from build123d import *

# Parameters (mm, degrees)
SKETCH1_W           = 20
SKETCH1_H           = 10
BOSS_EXTRUDE1_DEPTH = 20.5
SKETCH5_W           = 16
SKETCH5_H           = 12.5
BOSS_EXTRUDE2_DEPTH = 8
SKETCH2_R           = 5.1
CUT_EXTRUDE3_DEPTH  = 10
SKETCH6_W           = 5.5
SKETCH6_H           = 20
CUT_EXTRUDE4_DEPTH  = 8
SKETCH7_W           = 2.2
SKETCH7_H           = 2.2
CUT_EXTRUDE5_DEPTH  = 3
FILLET1_R           = 2


with BuildPart() as part:
    # Sketch1 → Boss-Extrude1 (new body)
    with BuildSketch(Plane.YZ):
        Rectangle(SKETCH1_W, SKETCH1_H)
    extrude(amount=BOSS_EXTRUDE1_DEPTH)

    # Sketch5 → Boss-Extrude2 (add)
    with BuildSketch(Plane(origin=(0, 0, 0), x_dir=(0, 1, 0), z_dir=(0, 0, 1))):
        with Locations((0, -12.25)):
            Rectangle(SKETCH5_W, SKETCH5_H)
    extrude(amount=BOSS_EXTRUDE2_DEPTH)

    # Sketch2 → Cut-Extrude3 (cut)
    with BuildSketch(Plane.YZ):
        Circle(SKETCH2_R)
    extrude(amount=CUT_EXTRUDE3_DEPTH, mode=Mode.SUBTRACT)

    # Sketch6 → Cut-Extrude4 (cut)
    with BuildSketch(Plane(origin=(0, 0, -5), x_dir=(1, 0, 0), z_dir=(0, 0, -1))):
        with Locations((17.75, 0)):
            Rectangle(SKETCH6_W, SKETCH6_H)
    extrude(amount=-CUT_EXTRUDE4_DEPTH, mode=Mode.SUBTRACT)

    # Sketch7 → Cut-Extrude5 (cut)
    with BuildSketch(Plane.YZ.offset(15)):
        with Locations((6, 0)):
            Rectangle(SKETCH7_W, SKETCH7_H)
        with Locations((-6, 0)):
            Rectangle(SKETCH7_W, SKETCH7_H)
    extrude(amount=-CUT_EXTRUDE5_DEPTH, mode=Mode.SUBTRACT)

    # Fillet1
    fillet1_edges = [part.edges().sort_by_distance(p)[0] for p in [
        (7.5, -10, -5),
        (7.5, 10, -5),
    ]]
    fillet(fillet1_edges, radius=FILLET1_R)


solid = part.part
Part model, mm, in its own coordinate system. A direction names the side the tool comes from. Give positions to 0.01 mm unless a question says otherwise; leave off trailing zeros. Loops run counter-clockwise (first coordinate to the right, second up) from the corner with the lowest first, then second, coordinate; pieces in that order, holes last. Notation, with made-up numbers: (40, 37) -> (62, 37) arc R19 ccw to (62, 60) -> close; hole circle Ø4 at (-23.75, -6.5). An arc over 180 degrees is marked (long way). Write each question's results on one line, items separated by ' | '. Start each with the question number.
Q1. Pin check, flat tips, straight feed: P1, Ø6, axis at x = 17, y = 1, coming from the -Z side; P2, Ø0.9, axis at y = 1.5, z = 6, coming from the +X side; P3, Ø4, axis at y = 2, z = 0, coming from the +X side; P4, Ø0.9, axis at y = 1.5, z = 7, coming from the -X side. Stop position of each tip, or through.
Q2. Pull direction Z, two halves, no side cores. Call faces 4 (the face through (14, -6, 1.1)), 5 (the face through (18, 0, 3)), 6 (the face through (12, 8, 6)): +Z half, -Z half, draft (parallel to the pull), parting line (faces both ways), or undercut.
Q3. Band-saw the part on D-D on x = 9.5. List the corners of the cut face in (y, z), plus the area to 3 significant figures.
Q4. Band-saw the part on B-B on z = 0. List the corners of the cut face in (x, y).
Q5. Wall check: L1, parallel to Y at x = 8, z = 0; L2, parallel to Z at x = 12.75, y = 5.25; L3, parallel to Y at x = 3.5, z = 1. Give the ranges that are in metal, low to high.
Q6. Which spindle directions (+Z, -Z, +X, -X, +Y, -Y) get a long thin tool onto all of the face, cutting with end or side? Do faces 1 (the face through (12, -8, 6)), 2 (the face through (14, -7.1, 0)), 3 (the face through (10, 0, 0)). Say none if no direction does.
Q7. Band-saw the part on C-C on y = 0. List the corners of the cut face in (x, z), plus the area to 3 significant figures.
Q8. Band-saw the part on A-A on x = 16.5. List the corners of the cut face in (y, z).
Results are:
1) P1: stops at z = -5 | P2: stops at x = 18.5 | P3: stops at x = 15 | P4: stops at x = 6
2) face 4: undercut | face 5: -Z half | face 6: draft
3) outline: (-10, -3) arc R2 ccw to (-8, -5) -> (-1, -5) arc R5.1 cw (long way) to (1, -5) -> (8, -5) arc R2 ccw to (10, -3) -> (10, 5) -> (8, 5) -> (8, 8) -> (-8, 8) -> (-8, 5) -> (-10, 5) -> close | area: 165 mm²
4) outline: (0, -10) -> (15, -10) -> (15, -7.1) -> (12, -7.1) -> (12, -4.9) -> (15, -4.9) -> (15, 4.9) -> (12, 4.9) -> (12, 7.1) -> (15, 7.1) -> (15, 10) -> (0, 10) -> (0, 5.1) -> (10, 5.1) -> (10, -5.1) -> (0, -5.1) -> close
5) L1: y = -10 to -5.1, 5.1 to 10 | L2: z = -5 to -1.1, 1.1 to 8 | L3: y = -10 to -5, 5 to 10
6) face 1: +Z, +X, -X, -Y | face 2: +X | face 3: -X
7) outline: (6, 5.1) -> (10, 5.1) -> (10, -5) -> (15, -5) -> (15, 3) -> (20.5, 3) -> (20.5, 5) -> (18.5, 5) -> (18.5, 8) -> (6, 8) -> close | area: 98.1 mm²
8) outline: (-10, 3) -> (10, 3) -> (10, 5) -> (8, 5) -> (8, 8) -> (-8, 8) -> (-8, 5) -> (-10, 5) -> close
